from build123d import *

# Parameters (mm, degrees)
F3_DEPTH = 2
F4_DEPTH = 0.5


with BuildPart() as f3:
    # F2 (on face) → F3 (new body)
    with BuildSketch(Plane(origin=(0, 0, 0), x_dir=(1, 0, 0), z_dir=(0, -0.7071067812, 0.7071067812))):
        Polygon((-14.9508744776, 21.5), (-36.4508744776, 0), (40.5491255224, 0), (19.0491255224, 21.5), (19.0491255224, 61.5), (-14.9508744776, 61.5), align=None)
    extrude(amount=F3_DEPTH)

    # F0 (on Top) → F4 (join)
    with BuildSketch(Plane.XY):
        Polygon((40.6194950176, 0), (-36.539348602, 0), (-36.4647228283, -14.9998143653), (-12.5346706987, -14.9998143653), (-12.5346706987, -20), (-7.3805049824, -20), (-7.3805049824, -14.9998143653), (12.6194950176, -14.9998143653), (12.6194950176, -20), (17.6194950176, -20), (17.6194950176, -15), (40.6194950176, -15), align=None)
    extrude(amount=F4_DEPTH)


solid = f3.part
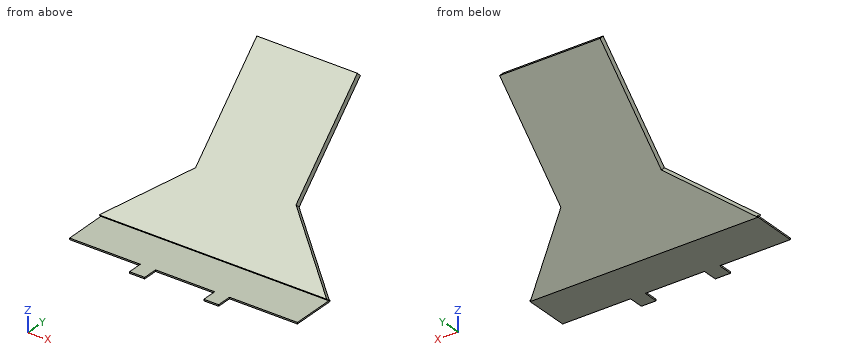
For this review, take the finished solid that the model builds, in its own axes (mm). Coordinates: 2 decimals unless noted, no trailing zeros. Loops run counter-clockwise (first coordinate to the right, second up) from the corner with the lowest first, then second, coordinate; pieces in that order, holes last. Notation, with made-up numbers: (84.5, 53.5) - (125.5, 53.5) arc R27 cw to (125.5, 78.5) - close; hole circle Ø3 at (-30.5, 85). An arc over 180 degrees is marked (long way). Return JSON: item names as keys, results as strings.
Item 1: Take a section at C-C (x = -31). Give the boundary of the cut face in (y, z).
Determined:
{"outline": "(-15, 0) - (0, 0) - (3.85, 3.85) - (2.44, 5.27) - (-1.41, 1.41) - (-0.5, 0.5) - (-15, 0.5) - close"}
Item 2: Take a section at B-B (z = 34). Give the boundary of the cut face in (x, y).
Determined:
{"outline": "(-14.95, 31.17) - (19.05, 31.17) - (19.05, 34) - (-14.95, 34) - close"}
Item 3: For line 1 (Z direction, x = 12.5, y = -4); line 2 (Z direction, x = 4, y = 23.5); line 3 (X direction, y = 25, z = 27), list the stretches that pass through material, from the lowest coordinate up.
Determined:
{"line 1": "z = 0 to 0.5", "line 2": "z = 23.5 to 26.33", "line 3": "x = -14.95 to 19.05"}
Item 4: Insertion check: pin 1 (3 mm diameter, centred on x = -7, y = 18.5, fed in from +Z); pin 2 (1 mm diameter, centred on x = 6, z = 12, fed in from +Y); pin 3 (0.6 mm diameter, centred on x = 2.5, z = 0.5, fed in from -Y). Each pin has a flat end and moves straight along its axis. Give the tip position at first contact, or say it passes through.
Determined:
{"pin 1": "stops at z = 22.83", "pin 2": "stops at y = 12.5", "pin 3": "stops at y = -15"}
Item 5: Take a section at A-A (x = 8.5). Give the boundary of the cut face in (y, z), then the cut area to 3 significant figures.
Determined:
{"outline": "(-15, 0) - (0, 0) - (43.49, 43.49) - (42.07, 44.9) - (-1.41, 1.41) - (-0.5, 0.5) - (-15, 0.5) - close", "area": "130 mm2"}
Item 6: Take a section at D-D (y = 36). Give the boundary of the cut face in (x, z).
Determined:
{"outline": "(-14.95, 36) - (19.05, 36) - (19.05, 38.83) - (-14.95, 38.83) - close"}
